Verification items for this drawing (mm, ordinates from the low corner). A direction names the side the tool comes from. Round coordinates to 2 decimals unless told otherwise and drop trailing zeros. Loops run counter-clockwise (first coordinate to the right, second up) from the corner with the lowest first, then second, coordinate; pieces in that order, holes last. Notation, with made-up numbers: (32, 11.5) - (69, 11.5) arc R24 cw to (69, 23.5) - close; hole circle Ø3 at (-21, 62). An arc over 180 degrees is marked (long way). Put each result on its own line as item: value.
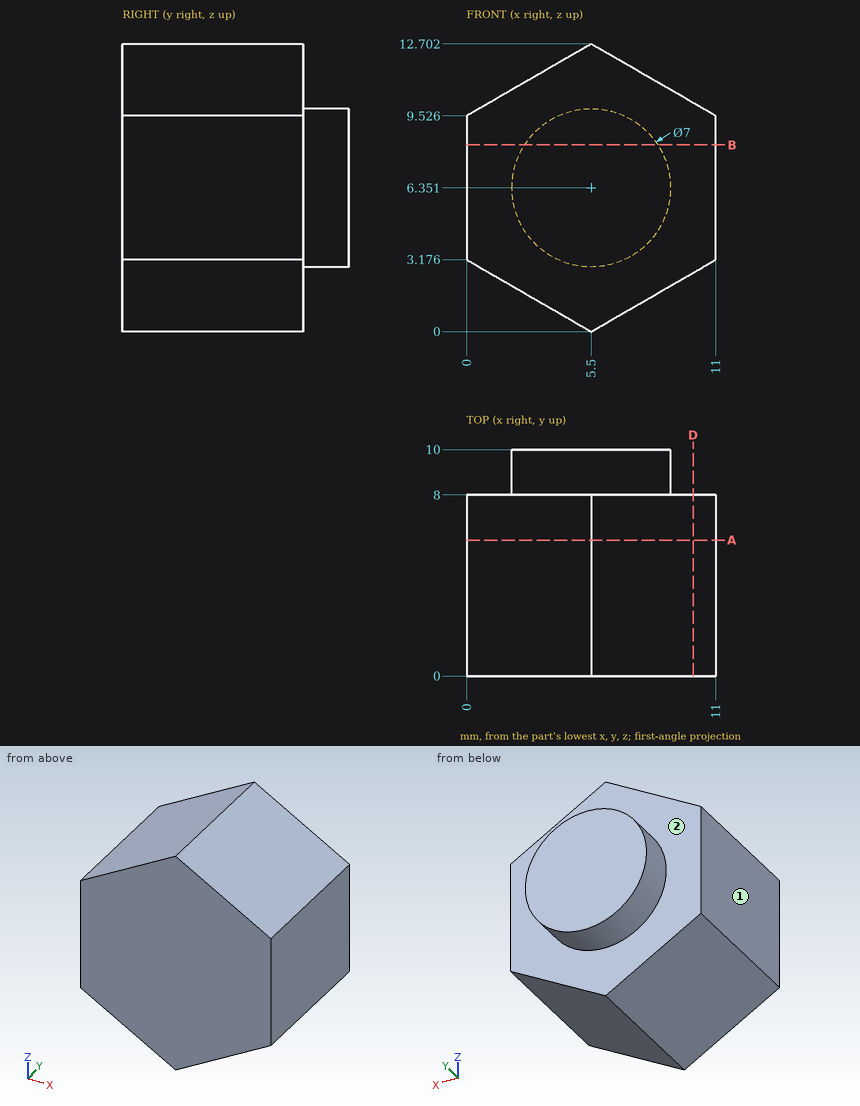
Item 1: Tool access check on the marked faces 1 and 2. Record the directions out of +Z, -Z, +X, -X, +Y, -Y that give a thin tool (end or side, any length) a straight path to the whole face; none if there is none.
Filled sheet:
face 1: +Z, -Z, -X, +Y, -Y
face 2: +Y
Item 2: Section check B-B on z = 8.25. Enter the section's corners in (x, y).
Filled sheet:
outline: (0, 0) - (11, 0) - (11, 8) - (8.44, 8) - (8.44, 10) - (2.56, 10) - (2.56, 8) - (0, 8) - close
Item 3: Section check D-D on x = 10. Enter the section's corners in (y, z).
Filled sheet:
outline: (0, 2.6) - (8, 2.6) - (8, 10.1) - (0, 10.1) - close
Item 4: Section check A-A on y = 6. Enter the section's corners in (x, z) (1 decimal).
Filled sheet:
outline: (0, 3.2) - (5.5, 0) - (11, 3.2) - (11, 9.5) - (5.5, 12.7) - (0, 9.5) - close
Item 5: Go/stop test with a flat-tipped pin: pin 1 (3 mm diameter, centred on x = 5.5, y = 6, fed in from +Z). Record where the tip stops, or that it passes through.
Filled sheet:
pin 1: z = 12.7
Item 6: Thickness scan on line 1 (X direction, y = 8.5, z = 6.5); line 2 (Y direction, x = 2.5, z = 10.25); line 3 (Z direction, x = 5.5, y = 9.5). Record the ranges inside material, lowest first. Write a range as from..to.
Filled sheet:
line 1: 2..9
line 2: 0..8
line 3: 2.85..9.85
